Part model, mm, in its own coordinate system. Face numbers are marked on the shaded views. A direction names the side the tool comes from. Give positions to 0.01 mm unless a question says otherwise; leave off trailing zeros. Loops run counter-clockwise (first coordinate to the right, second up) from the corner with the lowest first, then second, coordinate; pieces in that order, holes last. Notation, with made-up numbers: (-35, 24) -> (8, 24) arc R13 ccw to (8, 32) -> close; hole circle Ø1 at (44.25, 58). An arc over 180 degrees is marked (long way). One line per question, with ' | ' between items.
```python
from build123d import *

# Parameters (mm, degrees)
SKETCH1_W           = 50
SKETCH1_H           = 50
BOSS_EXTRUDE1_DEPTH = 5
LOFT1_START         = -7.5
LOFT1_DEPTH         = 15
SKETCH7_R           = 3.15
CUT_EXTRUDE1_DEPTH  = 39.405728778


# Read off the part's stored shape, not the designer's step: Loft1
with BuildPart() as part:
    # Sketch1 → Boss-Extrude1 (new body)
    with BuildSketch(Plane(origin=(0, 0, 0), x_dir=(1, 0, 0), z_dir=(0, 1, 0))):
        Rectangle(SKETCH1_W, SKETCH1_H)
    extrude(amount=BOSS_EXTRUDE1_DEPTH)

    # Loft1 outline → Loft1 (add)
    with BuildSketch(Plane.XY.offset(LOFT1_START)):
        with BuildLine():
            add(Edge.make_bspline(
                [(2.5, 15), (2.5, 10.833333333), (6.25, 7.916666667), (10, 5)],
                knots=[0, 0, 0, 0, 1, 1, 1, 1], degree=3))
            Line((2.5, 15), (-2.5, 15))
            add(Edge.make_bspline(
                [(-2.5, 15), (-2.5, 10.833333333), (-6.25, 7.916666667), (-10, 5)],
                knots=[0, 0, 0, 0, 1, 1, 1, 1], degree=3))
            Line((-10, 5), (10, 5))
        make_face()
    extrude(amount=LOFT1_DEPTH)

    # Sketch7 → Cut-Extrude1 (cut, through all)
    with BuildSketch(Plane(origin=(0, 0, 0), x_dir=(-1, 0, 0), z_dir=(0, -1, 0))):
        with Locations(Location((21, -21, 0), (0, 0, 90))):
            Circle(SKETCH7_R)
        with Locations(Location((-21, -21, 0), (0, 0, 90))):
            Circle(SKETCH7_R)
        with Locations(Location((-21, 21, 0), (0, 0, 90))):
            Circle(SKETCH7_R)
        with Locations(Location((21, 21, 0), (0, 0, 90))):
            Circle(SKETCH7_R)
    extrude(amount=-CUT_EXTRUDE1_DEPTH, mode=Mode.SUBTRACT)


solid = part.part
```
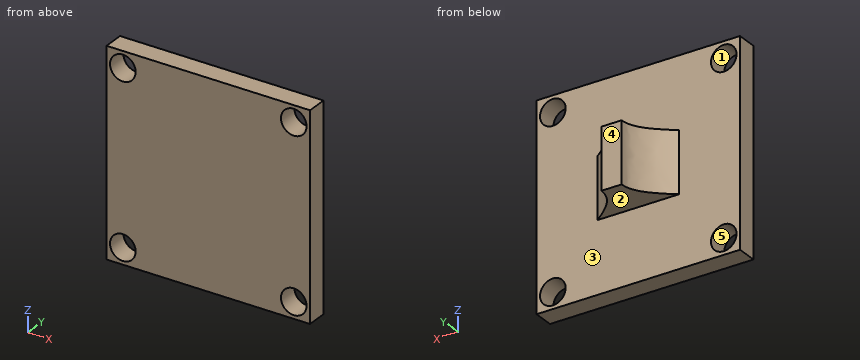
1) Pull direction X, two halves, no side cores. Call the marked faces 4 and 5: pulls with the +X half, pulls with the -X half, needs draft (parallel to the pull), parting line crosses it, or undercut.
Found:
face 4: needs draft | face 5: undercut
2) Saw through at D-D (z = 12). Give the cut face in (x, y).
Found:
outline: (-25, 0) -> (25, 0) -> (25, 5) -> (-25, 5) -> close
3) Tool access for the marked faces 1, 2 and 3: list every direction of +Z, -Z, +X, -X, +Y, -Y with a clear straight run to the whole face (end or side of a thin tool).
Found:
face 1: +Y, -Y | face 2: -Z, +X, -X, +Y | face 3: +Y
4) Saw through at B-B (y = 2). Give the cut face in (x, z).
Found:
outline: (-25, -25) -> (25, -25) -> (25, 25) -> (-25, 25) -> close; hole circle Ø6.3 at (-21, -21); hole circle Ø6.3 at (-21, 21); hole circle Ø6.3 at (21, -21); hole circle Ø6.3 at (21, 21)
5) Saw through at A-A (x = 21). Give the cut face in (y, z).
Found:
outline: (0, -25) -> (5, -25) -> (5, -24.15) -> (0, -24.15) -> close; (0, -17.85) -> (5, -17.85) -> (5, 17.85) -> (0, 17.85) -> close; (0, 24.15) -> (5, 24.15) -> (5, 25) -> (0, 25) -> close
6) Saw through at C-C (z = -21). Give the cut face in (x, y).
Found:
outline: (-25, 0) -> (-24.15, 0) -> (-24.15, 5) -> (-25, 5) -> close; (-17.85, 0) -> (17.85, 0) -> (17.85, 5) -> (-17.85, 5) -> close; (24.15, 0) -> (25, 0) -> (25, 5) -> (24.15, 5) -> close
7) Drill centre lines: line 1 (X direction, y = 1.6, z = -21); line 2 (Y direction, x = -4.5, z = -15); line 3 (Z direction, x = 1, y = 10.5). Where is each one in solid material? Low to high.
Found:
line 1: -25 to -24.15, -17.85 to 17.85, 24.15 to 25 | line 2: 0 to 5 | line 3: -7.5 to 7.5
8) Pin check, flat tips, straight feed: P1, Ø5.5, axis at x = 21, z = 21, coming from the -Y side; P2, Ø1, axis at y = 13.5, z = 5.5, coming from the -X side; P3, Ø2, axis at x = -12, z = 18.5, coming from the +Y side; P4, Ø5, axis at x = 0, y = 8, coming from the +Z side. Stop position of each tip, or through.
Found:
P1: through | P2: x = -2.8 | P3: y = 5 | P4: z = 7.5
